For this review, take the finished solid that the model builds, in its own axes (mm). Face numbers are marked on the shaded views. Give positions to 0.01 mm unless a question says otherwise; leave off trailing zeros. Loops run counter-clockwise (first coordinate to the right, second up) from the corner with the lowest first, then second, coordinate; pieces in that order, holes last. Notation, with made-up numbers: (58, 57) - (82, 57) arc R22 cw to (82, 94) - close; hole circle Ø9 at (32.5, -1). An arc over 180 degrees is marked (long way). Answer as CSV lines item,"result".
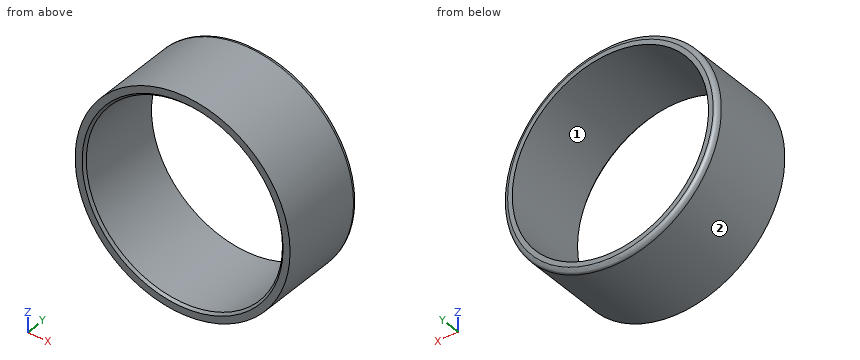
from build123d import *

# Parameters (mm, degrees)
SKETCH1_R           = 23
SKETCH1_R_2         = 21
EXTRUDE_THIN1_DEPTH = 19
FILLET1_R           = 1
CHAMFER1_SIZE       = 0.5


with BuildPart() as part:
    # Sketch1 → Extrude-Thin1 (new body)
    with BuildSketch(Plane(origin=(0, 0, 0), x_dir=(1, 0, 0), z_dir=(0, 1, 0))):
        Circle(SKETCH1_R)
        Circle(SKETCH1_R_2, mode=Mode.SUBTRACT)
    extrude(amount=EXTRUDE_THIN1_DEPTH)

    # Fillet1
    fillet1_edges = [part.edges().sort_by_distance(p)[0] for p in [
        (-23, 19, 0),
    ]]
    fillet(fillet1_edges, radius=FILLET1_R)

    # Chamfer1
    chamfer1_edges = [part.edges().sort_by_distance(p)[0] for p in [
        (-21, 0, 0),
    ]]
    chamfer(chamfer1_edges, length=CHAMFER1_SIZE)


solid = part.part
1) Consider section C-C on y = 7.75. Write out the cut boundary in (x, z).
From the geometry:
outline,"circle Ø46 at (0, 0); hole circle Ø42 at (0, 0)"
2) Consider section B-B on z = 0. Write out the cut boundary in (x, y), and give its area (3 significant figures).
From the geometry:
outline,"(-23, 0) - (-21.5, 0) - (-21, 0.5) - (-21, 19) - (-22, 19) arc R1 ccw to (-23, 18) - close; (21, 0.5) - (21.5, 0) - (23, 0) - (23, 18) arc R1 ccw to (22, 19) - (21, 19) - close"
area,"75.3 mm^2"
3) Consider section A-A on x = 0. Write out the cut boundary in (y, z), and give its area (3 significant figures).
From the geometry:
outline,"(0, -23) - (18, -23) arc R1 ccw to (19, -22) - (19, -21) - (0.5, -21) - (0, -21.5) - close; (0, 21.5) - (0.5, 21) - (19, 21) - (19, 22) arc R1 ccw to (18, 23) - (0, 23) - close"
area,"75.3 mm^2"
4) Wall thickness on line 1 (Z direction, x = 0, y = 14.25); line 2 (Z direction, x = 14, y = 14.5): over which ranges is each line inside the solid? List them lowest first. Write a range as from..to.
From the geometry:
line 1,"z = -23..-21, 21..23"
line 2,"z = -18.25..-15.65, 15.65..18.25"
5) Insertion check: P1, Ø2, axis at x = -4, y = 12, coming from the +Z side; P2, Ø1.5, axis at x = 9.5, y = 13, coming from the +Z side; P3, Ø10, axis at y = 17, z = 16, coming from the +X side. Each pin has a flat end and moves straight along its axis. Give the tip position at first contact, or say it passes through.
From the geometry:
P1,"stops at z = 22.8"
P2,"stops at z = 21.27"
P3,"stops at x = 20.2"
6) Draft analysis for pull direction Z (two halves, no side actions). For the marked faces 1 and 2, state which applies: pulls with the +Z half, pulls with the -Z half, needs draft (parallel to the pull), parting line crosses it, or undercut.
From the geometry:
face 1,"undercut"
face 2,"parting line crosses it"
